For this review, take the finished solid that the model builds, in its own axes (mm). Face numbers are marked on the shaded views. A direction names the side the tool comes from. Give positions to 0.01 mm unless a question says otherwise; leave off trailing zeros. Order: outer loops, then holes, each group sorted by start corner. A loop starts at its lowest first (then second) coordinate and runs counter-clockwise, first axis right, second up. Notation, with made-up numbers: M -20.5,-23.5 L 27.5,-23.5 A24 ccw 27.5,-13.5 Z; hole C -18,-7 d8. An arc over 180 degrees is marked long. Use CSV: the item, a comma, the result in double quotes. Start each with the question number.
(1) Tool access review of the marked faces 1, 2, 3, 4 and 5: name each direction out of +Z, -Z, +X, -X, +Y, -Y from which nothing blocks a thin tool from reaching the whole face with its end or side.
(2) Consider section B-B (z = 12.25). Write out the cut boundary in (x, y), and give its area (4 significant figures).
(3) Wall thickness on L1, parallel to Z at x = -2.75, y = 21.5; L2, parallel to Y at x = -3.75, z = 3; L3, parallel to X at y = 17.5, z = 2: over which ranges is each line inside the solid? List them lowest first. Write a range as from..to.
(4) Consider section D-D (z = 4). Write out the cut boundary in (x, y).
(5) Consider section C-C (y = 20.5). Write out the cut boundary in (x, z).
(6) Consider section A-A (x = -0.75). Write out the cut boundary in (y, z) (3 decimals), and give its area (3 significant figures).
(7) Clearance check with flat-ended pins moving along their axes: P1, Ø1.2, axis at x = -1, z = -13, coming from the -Y side; P2, Ø5, axis at y = 20.5, z = -12.5, coming from the -X side; P3, Ø1.2, axis at x = -1, z = -11, coming from the +Y side. State where each tip first meets the part, or that it passes through.
(8) Draft analysis for pull direction Y (two halves, no side actions). For the marked faces 6, 7, 8 and 9, state which applies: pulls with the +Y half, pulls with the -Y half, needs draft (parallel to the pull), parting line crosses it, or undercut.
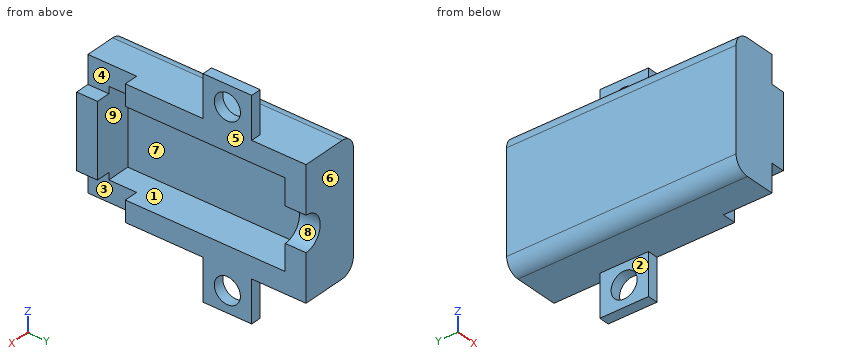
```python
from build123d import *

# Parameters (mm, degrees)
SKETCH1_W           = 16.7
SKETCH1_H           = 18.5
BOSS_EXTRUDE1_DEPTH = 3
SKETCH2_W           = 16.7
SKETCH2_H           = 18.5
SKETCH2_W_2         = 10.7
SKETCH2_H_2         = 12.5
BOSS_EXTRUDE2_DEPTH = 27
SKETCH7_W           = 4
SKETCH7_H           = 8
CUT_EXTRUDE1_DEPTH  = 7
SKETCH9_W           = 16.7
SKETCH9_H           = 18.5
BOSS_EXTRUDE3_DEPTH = 3
SKETCH10_R          = 2.5
CUT_EXTRUDE2_DEPTH  = 3
FILLET1_R           = 2
SKETCH11_W          = 3
SKETCH11_H          = 7
BOSS_EXTRUDE4_DEPTH = 6
SKETCH12_R          = 1.875
CUT_EXTRUDE3_DEPTH  = 6
CUT_EXTRUDE4_START  = -33
CUT_EXTRUDE4_DEPTH  = 33


# Read off the part's stored shape, not the designer's step: Cut-Extrude4
with BuildPart() as part:
    # Sketch1 → Boss-Extrude1 (new body)
    with BuildSketch(Plane(origin=(0, 0, 0), x_dir=(1, 0, 0), z_dir=(0, 1, 0))):
        Rectangle(SKETCH1_W, SKETCH1_H)
    extrude(amount=BOSS_EXTRUDE1_DEPTH)

    # Sketch2 → Boss-Extrude2 (add)
    with BuildSketch(Plane(origin=(0, 3, 0), x_dir=(1, 0, 0), z_dir=(0, 1, 0))):
        Rectangle(SKETCH2_W, SKETCH2_H)
        Rectangle(SKETCH2_W_2, SKETCH2_H_2, mode=Mode.SUBTRACT)
    extrude(amount=BOSS_EXTRUDE2_DEPTH)

    # Sketch7 → Cut-Extrude1 (cut)
    with BuildSketch(Plane.XZ):
        with Locations((0, 9.25)):
            Rectangle(SKETCH7_W, SKETCH7_H)
        with Locations((0, -9.25)):
            Rectangle(SKETCH7_W, SKETCH7_H)
    extrude(amount=-CUT_EXTRUDE1_DEPTH, mode=Mode.SUBTRACT)

    # Sketch9 → Boss-Extrude3 (add)
    with BuildSketch(Plane(origin=(0, 30, 0), x_dir=(1, 0, 0), z_dir=(0, 1, 0))):
        Rectangle(SKETCH9_W, SKETCH9_H)
    extrude(amount=BOSS_EXTRUDE3_DEPTH)

    # Sketch10 → Cut-Extrude2 (cut)
    with BuildSketch(Plane(origin=(0, 33, 0), x_dir=(1, 0, 0), z_dir=(0, 1, 0))):
        with Locations(Location((0, 0, 0), (0, 0, 270))):
            Circle(SKETCH10_R)
    extrude(amount=-CUT_EXTRUDE2_DEPTH, mode=Mode.SUBTRACT)

    # Fillet1
    fillet1_edges = [part.edges().sort_by_distance(p)[0] for p in [
        (8.35, 16.5, 9.25),
        (-8.35, 16.5, 9.25),
        (-8.35, 16.5, -9.25),
        (8.35, 16.5, -9.25),
    ]]
    fillet(fillet1_edges, radius=FILLET1_R)

    # Sketch11 → Boss-Extrude4 (add)
    with BuildSketch(Plane.XY.offset(9.25)):
        with Locations((0, 21.679413475)):
            Rectangle(SKETCH11_W, SKETCH11_H)
    boss_extrude4 = extrude(amount=BOSS_EXTRUDE4_DEPTH)

    # Sketch12 → Cut-Extrude3 (cut)
    with BuildSketch(Plane(origin=(1.5, 0, 0), x_dir=(0, 0, -1), z_dir=(1, 0, 0))):
        with Locations(Location((-12.25, 21.679413475, 0), (0, 0, 90))):
            Circle(SKETCH12_R)
    cut_extrude3 = extrude(amount=-CUT_EXTRUDE3_DEPTH, mode=Mode.SUBTRACT)

    # Mirror1: Boss-Extrude4, Cut-Extrude3 across plane
    add(boss_extrude4.mirror(Plane.XY))
    add(cut_extrude3.mirror(Plane.XY), mode=Mode.SUBTRACT)

    # Cut-Extrude4 outline → Cut-Extrude4 (cut)
    with BuildSketch(Plane(origin=(0, 33, 0), x_dir=(1, 0, 0), z_dir=(0, 1, 0)).offset(CUT_EXTRUDE4_START)):
        with BuildLine():
            Line((0, -15.25), (1.5, -15.25))
            Line((1.5, -15.25), (1.5, -9.25))
            Line((1.5, -9.25), (6.35, -9.25))
            ThreePointArc((6.35, -9.25), (7.764213562, -8.664213562), (8.35, -7.25))
            Line((8.35, -7.25), (8.35, 7.25))
            ThreePointArc((8.35, 7.25), (7.764213562, 8.664213562), (6.35, 9.25))
            Line((6.35, 9.25), (1.5, 9.25))
            Line((1.5, 9.25), (1.5, 15.25))
            Line((1.5, 15.25), (0, 15.25))
            Line((0, 15.25), (0, -15.25))
        make_face()
    extrude(amount=CUT_EXTRUDE4_DEPTH, mode=Mode.SUBTRACT)


solid = part.part
```
Check result:
1,face 1,"+X"
1,face 2,"-Z, -X, +Y, -Y"
1,face 3,"-Z, +X, -Y"
1,face 4,"+Z, +X, -Y"
1,face 5,"+Z, -Z, +X, +Y, -Y"
2,outline,"M -1.5,18.18 L 0,18.18 L 0,19.8 L -1.5,19.8 Z; M -1.5,23.55 L 0,23.55 L 0,25.18 L -1.5,25.18 Z"
2,area,"4.875 mm^2"
3,L1,"z = -9.25..-6.25, 6.25..9.25"
3,L2,"y = 0..3, 30..33"
3,L3,"x = -8.35..-5.35"
4,outline,"M -8.35,0 L 0,0 L 0,3 L -5.35,3 L -5.35,30 L 0,30 L 0,33 L -8.35,33 Z"
5,outline,"M -8.35,-7.25 A2 ccw -6.35,-9.25 L -1.5,-9.25 L -1.5,-10.79 L 0,-10.79 L 0,-6.25 L -5.35,-6.25 L -5.35,6.25 L 0,6.25 L 0,10.79 L -1.5,10.79 L -1.5,9.25 L -6.35,9.25 A2 ccw -8.35,7.25 Z; M -1.5,-15.25 L 0,-15.25 L 0,-13.71 L -1.5,-13.71 Z; M -1.5,13.71 L 0,13.71 L 0,15.25 L -1.5,15.25 Z"
6,outline,"M 0,-5.25 L 3,-5.25 L 3,5.25 L 0,5.25 Z; M 7,-9.25 L 18.179,-9.25 L 18.179,-15.25 L 25.179,-15.25 L 25.179,-9.25 L 33,-9.25 L 33,-2.385 L 30,-2.385 L 30,-6.25 L 7,-6.25 Z; M 7,6.25 L 30,6.25 L 30,2.385 L 33,2.385 L 33,9.25 L 25.179,9.25 L 25.179,15.25 L 18.179,15.25 L 18.179,9.25 L 7,9.25 Z; hole C 21.679,-12.25 d3.75; hole C 21.679,12.25 d3.75"
6,area,"273 mm^2"
7,P1,"stops at y = 18.18"
7,P2,"stops at x = -1.5"
7,P3,"stops at y = 25.18"
8,face 6,"pulls with the +Y half"
8,face 7,"undercut"
8,face 8,"needs draft"
8,face 9,"undercut"
